```python
from build123d import *

# Parameters (mm, degrees)
CAP_OD26_ID8_THICKNESS2_PROFILE_R   = 13
CAP_OD26_ID8_THICKNESS2_PROFILE_R_2 = 4
CAP_OD26_ID8_THICKNESS2_DEPTH       = 2
FOUR_M2_CAPTURE_HOLES_START         = -50
FOUR_M2_CAPTURE_HOLES_PROFILE_R     = 1.15
FOUR_M2_CAPTURE_HOLES_DEPTH         = 69.493242009
LOW_PROFILE_HEAD_SEATS_R            = 2.1
HEAD_RECESS_DEPTH0P55_DEPTH         = 0.55


with BuildPart() as part:
    # Cap_OD26_ID8_thickness2_profile → Cap_OD26_ID8_thickness2 (new body)
    with BuildSketch(Plane.XY):
        Circle(CAP_OD26_ID8_THICKNESS2_PROFILE_R)
        Circle(CAP_OD26_ID8_THICKNESS2_PROFILE_R_2, mode=Mode.SUBTRACT)
    extrude(amount=CAP_OD26_ID8_THICKNESS2_DEPTH)

    # Four_M2_capture_holes_profile → Four_M2_capture_holes (cut, through all)
    with BuildSketch(Plane.XY.offset(FOUR_M2_CAPTURE_HOLES_START)):
        with Locations((7, 7)):
            Circle(FOUR_M2_CAPTURE_HOLES_PROFILE_R)
        with Locations((-7, 7)):
            Circle(FOUR_M2_CAPTURE_HOLES_PROFILE_R)
        with Locations((-7, -7)):
            Circle(FOUR_M2_CAPTURE_HOLES_PROFILE_R)
        with Locations((7, -7)):
            Circle(FOUR_M2_CAPTURE_HOLES_PROFILE_R)
    extrude(amount=FOUR_M2_CAPTURE_HOLES_DEPTH, mode=Mode.SUBTRACT)

    # Low_profile_head_seats → Head_recess_depth0p55 (cut)
    with BuildSketch(Plane.XY):
        with Locations((7, 7)):
            Circle(LOW_PROFILE_HEAD_SEATS_R)
        with Locations((-7, 7)):
            Circle(LOW_PROFILE_HEAD_SEATS_R)
        with Locations((-7, -7)):
            Circle(LOW_PROFILE_HEAD_SEATS_R)
        with Locations((7, -7)):
            Circle(LOW_PROFILE_HEAD_SEATS_R)
    extrude(amount=HEAD_RECESS_DEPTH0P55_DEPTH, mode=Mode.SUBTRACT)


solid = part.part
```
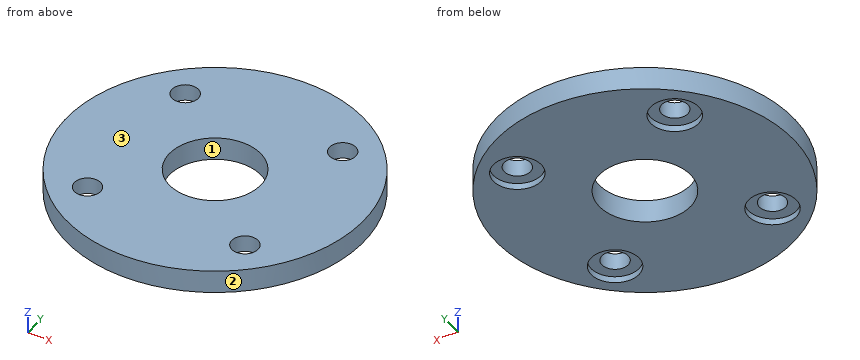
Source: CAD feature listing. Evaluate the final solid. Frame: model axes, mm. Face numbers are marked on the shaded views. Round coordinates to 2 decimals unless told otherwise and drop trailing zeros. Write each loop counter-clockwise with the first axis right and the second up, starting at its lowest first coordinate (ties: lowest second). Pieces come first, ordered by that corner, then holes. Notation, with made-up numbers: M -33,-12.5 L -2,-12.5 A12 cw -2,2.5 Z; hole C 7,-39 d3. An arc over 180 degrees is marked long. Answer as a JSON object with one key per item and string values. Group by question number.
(1) Mould query, pull axis Y, two halves, no side actions, for the marked faces 1, 2 and 3. Classes: +Y half, -Y half, draft (parallel to the pull), parting line (faces both ways), or undercut.
(2) Ray query, line 1 (X direction, y = 7, z = 1.25); line 2 (Y direction, x = 7, z = 0.45). Return the intervals inside material, ascending. Write a range as [from, to].
(3) Section query A-A on z = 0.85. Output: boundary loops of the cut face in (x, y).
(4) Section query B-B on y = 7. Output: boundary loops of the cut face in (x, z), then the cut area to 3 significant figures.
(5) First-contact query: pin 1 (3 mm diameter, centred on x = -7, y = 7, fed in from -Z); pin 2 (6.5 mm diameter, centred on x = 0, y = 0, fed in from +Z). Flat tips, straight axial feed; report the tip coordinate or a pass-through.
(6) Section query D-D on y = -1. Output: boundary loops of the cut face in (x, z).
Computed values:
{
 "1": {"face 1": "undercut", "face 2": "parting line", "face 3": "draft"},
 "2": {"line 1": "[-10.95, -8.15], [-5.85, 5.85], [8.15, 10.95]", "line 2": "[-10.95, -9.1], [-4.9, 4.9], [9.1, 10.95]"},
 "3": {"outline": "C 0,0 d26; hole C -7,-7 d2.3; hole C -7,7 d2.3; hole C 0,0 d8; hole C 7,-7 d2.3; hole C 7,7 d2.3"},
 "4": {"outline": "M -10.95,0 L -9.1,0 L -9.1,0.55 L -8.15,0.55 L -8.15,2 L -10.95,2 Z; M -5.85,0.55 L -4.9,0.55 L -4.9,0 L 4.9,0 L 4.9,0.55 L 5.85,0.55 L 5.85,2 L -5.85,2 Z; M 8.15,0.55 L 9.1,0.55 L 9.1,0 L 10.95,0 L 10.95,2 L 8.15,2 Z", "area": "32.5 mm^2"},
 "5": {"pin 1": "z = 0.55", "pin 2": "through"},
 "6": {"outline": "M -12.96,0 L -3.87,0 L -3.87,2 L -12.96,2 Z; M 3.87,0 L 12.96,0 L 12.96,2 L 3.87,2 Z"}
}
